Check sheet for the modelled part. Datum: model origin and axes. Units: mm. A direction names the side the tool comes from. Round coordinates to 2 decimals unless told otherwise and drop trailing zeros. Order: outer loops, then holes, each group sorted by start corner. A loop starts at its lowest first (then second) coordinate and runs counter-clockwise, first axis right, second up. Notation, with made-up numbers: (73, -10) -> (85, -10) arc R32 ccw to (85, 24) -> close; hole circle Ø10 at (34, -32.5). An arc over 180 degrees is marked (long way). Answer in a Markdown table with one row per item.
from build123d import *

# Parameters (mm, degrees)
F0_W     = 22.224892
F0_H     = 30.376296
F1_DEPTH = 25.4
F2_R     = 14.832934
F3_DEPTH = 25.401


with BuildPart() as f1:
    # F0 (on Front) → F1 (new body)
    with BuildSketch(Plane.XZ):
        Polygon((-60.305666, 60.30567), (-118.531823, 60.30567), (-118.531823, -34.93569), (-60.305666, -34.93569), (-60.305666, -25.506545), (-60.305666, 29.929374), align=None)
        Polygon((-38.080774, 29.929374), (-60.305666, 29.929374), (-60.305666, -25.506545), (-15.796112, -25.506545), (-15.796112, 29.929374), align=None)
        with Locations((-49.19322, 45.117522)):
            Rectangle(F0_W, F0_H)
    extrude(amount=F1_DEPTH)

    # F2 (on Front) → F3 (cut, through all)
    with BuildSketch(Plane.XZ):
        with Locations((-89.834586, 41.88443)):
            Circle(F2_R)
    extrude(amount=F3_DEPTH, mode=Mode.SUBTRACT)


solid = f1.part
Item 1: Scan lines: line 1 (Z direction, x = -90, y = -17); line 2 (Z direction, x = -53.5, y = -23.5); line 3 (X direction, y = -1, z = -28). Record each from-to range of solid material in increasing order. Write a range as [from, to].
Result sheet:
| item | result |
|---|---|
| line 1 | z = [-34.94, 27.05], [56.72, 60.31] |
| line 2 | z = [-25.51, 60.31] |
| line 3 | x = [-118.53, -60.31] |
Item 2: Cross-section at C-C (x = -94). Record the boundary of the cut face in (y, z).
Result sheet:
| item | result |
|---|---|
| outline | (-25.4, -34.94) -> (0, -34.94) -> (0, 27.65) -> (-25.4, 27.65) -> close; (-25.4, 56.12) -> (0, 56.12) -> (0, 60.31) -> (-25.4, 60.31) -> close |
Item 3: Depth check by flat-ended pin: P1, Ø11, axis at x = -27.5, y = -15.5, coming from the +Z side; P2, Ø10.5, axis at y = -7.5, z = -31.5, coming from the +X side; P3, Ø1.5, axis at x = -52, y = -12, coming from the -Z side. Enter the tip coordinate at first touch or a pass-through.
Result sheet:
| item | result |
|---|---|
| P1 | stops at z = 29.93 |
| P2 | stops at x = -60.31 |
| P3 | stops at z = -25.51 |
Item 4: Cross-section at B-B (y = -20). Record the boundary of the cut face in (x, z).
Result sheet:
| item | result |
|---|---|
| outline | (-118.53, -34.94) -> (-60.31, -34.94) -> (-60.31, -25.51) -> (-15.8, -25.51) -> (-15.8, 29.93) -> (-38.08, 29.93) -> (-38.08, 60.31) -> (-118.53, 60.31) -> close; hole circle Ø29.67 at (-89.83, 41.88) |
Item 5: Cross-section at A-A (z = 33.5). Record the boundary of the cut face in (x, y), and give its area (3 significant figures).
Result sheet:
| item | result |
|---|---|
| outline | (-118.53, -25.4) -> (-102.07, -25.4) -> (-102.07, 0) -> (-118.53, 0) -> close; (-77.6, -25.4) -> (-38.08, -25.4) -> (-38.08, 0) -> (-77.6, 0) -> close |
| area | 1,420 mm^2 |
Item 6: Mould release check, pull along X, two halves, no side actions. Record for faces 4 (the flat face through (-68, 0, 13)), 5 (the flat face through (-60.306, -13, -30)), 6 (the cylindrical face through (-75.687, -12.522, 46.34)): pulls with the +X half, pulls with the -X half, needs draft (parallel to the pull), parting line crosses it, or undercut.
Result sheet:
| item | result |
|---|---|
| face 4 | needs draft |
| face 5 | pulls with the +X half |
| face 6 | undercut |
Item 7: Cross-section at D-D (x = -52.5). Record the boundary of the cut face in (y, z).
Result sheet:
| item | result |
|---|---|
| outline | (-25.4, -25.51) -> (0, -25.51) -> (0, 60.31) -> (-25.4, 60.31) -> close |
Item 8: Set-up check for faces 1 (the flat face through (-27, -13, 29.929)), 2 (the flat face through (-38, -13, -25.507)), 3 (the flat face through (-15.796, -13, 2)): record each of +Z, -Z, +X, -X, +Y, -Y from which the full face is reachable in a straight line by a thin tool's end or side.
Result sheet:
| item | result |
|---|---|
| face 1 | +Z, +X, +Y, -Y |
| face 2 | -Z, +X, +Y, -Y |
| face 3 | +Z, -Z, +X, +Y, -Y |
